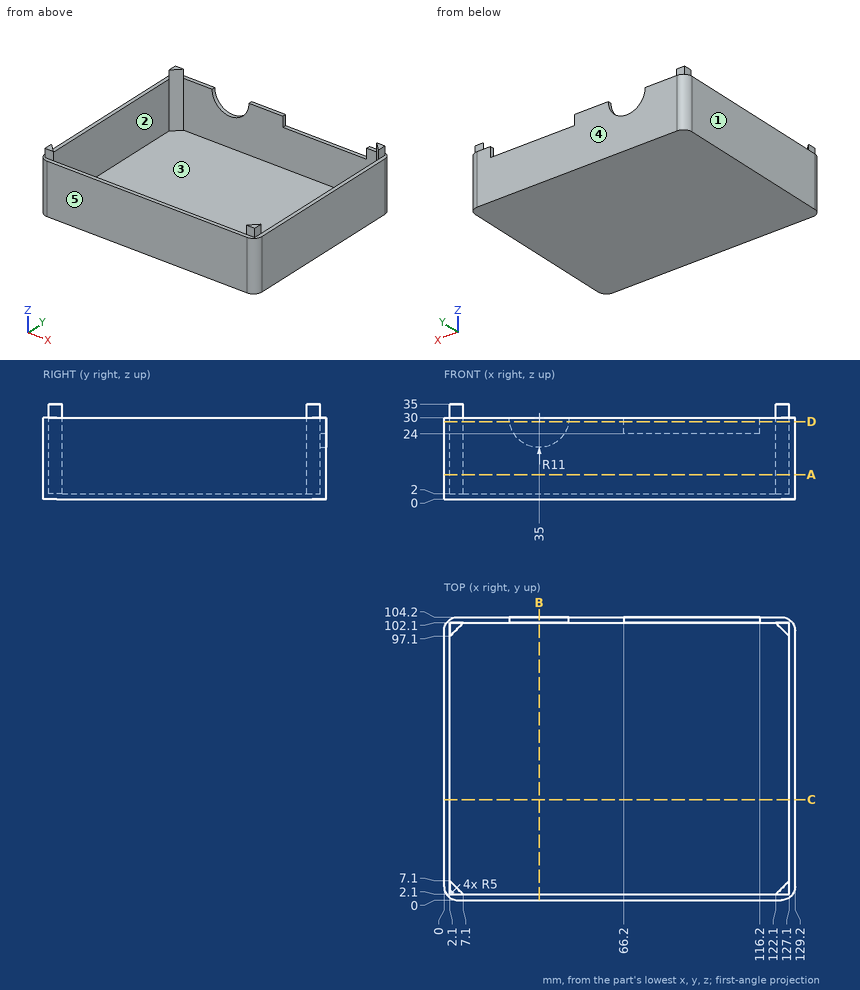
Study the drawing (mm; zero at the part's minimum x, y, z) and answer. A direction names the side the tool comes from. Give positions to 0.01 mm unless a question says otherwise; leave off trailing zeros. Write each loop counter-clockwise with the first axis right and the second up, starting at its lowest first coordinate (ties: lowest second). Pieces come first, ordered by that corner, then holes. Notation, with made-up numbers: (-26, 0) -> (-10, 0) arc R25 cw to (-10, 21) -> close; hole circle Ø3 at (-30.5, 35.25). An arc over 180 degrees is marked (long way). Answer as a JSON object with one key per item and string values. Group by question number.
1) Consider L1, parallel to X at y = 55.5, z = 11; L2, parallel to Y at x = 73, z = 19.5; L3, parallel to Z at x = 58.5, y = 5. Determine where each line is inside the solid, lowest interval first. Write a range as from..to.
2) Each of these flat-tipped pins is pushed along its axis until it touches: P1, Ø1.7, axis at x = 51.5, y = 103, coming from the +Z side; P2, Ø1.5, axis at x = 5, z = 32.5, coming from the +Y side; P3, Ø2.5, axis at y = 100.5, z = 33.5, coming from the +X side. Where does it stop, or does it pass through?
3) Find section B-B (x = 35). Write down the section's boundary in (y, z), and give its area (3 significant figures).
4) The mould has two halves that part along Y. Classify the marked faces 3, 4 and 5: +Y half, -Y half, draft (parallel to the pull), parting line (faces both ways), or undercut.
5) Find section A-A (z = 9). Write down the section's boundary in (x, y), and give its area (3 significant figures).
6) A tool of negligible diameter and unlimited length cuts with its end or side. For the marked faces 1 and 2, from which of +Z, -Z, +X, -X, +Y, -Y can it reach the whole face along a straight path? Write none if from no direction.
7) Find section D-D (z = 28.5). Write down the section's boundary in (x, y), and give its area (3 significant figures).
8) Find section C-C (y = 37). Write down the section's boundary in (x, z), and give its area (3 significant figures).
Values follow:
{
 "1": {"L1": "x = 0..2.1, 127.1..129.2", "L2": "y = 0..2.1, 102.1..104.2", "L3": "z = 0..2"},
 "2": {"P1": "stops at z = 30", "P2": "stops at y = 102.1", "P3": "stops at x = 127.1"},
 "3": {"outline": "(0, 0) -> (104.2, 0) -> (104.2, 19) -> (102.1, 19) -> (102.1, 2) -> (2.1, 2) -> (2.1, 30) -> (0, 30) -> close", "area": "303 mm2"},
 "4": {"face 3": "undercut", "face 4": "+Y half", "face 5": "-Y half"},
 "5": {"outline": "(0, 5) arc R5 ccw to (5, 0) -> (124.2, 0) arc R5 ccw to (129.2, 5) -> (129.2, 99.2) arc R5 ccw to (124.2, 104.2) -> (5, 104.2) arc R5 ccw to (0, 99.2) -> close; hole (2.1, 7.1) -> (7.1, 2.1) -> (122.1, 2.1) -> (127.1, 7.1) -> (127.1, 97.1) -> (122.1, 102.1) -> (7.1, 102.1) -> (2.1, 97.1) -> close", "area": "991 mm2"},
 "6": {"face 1": "+Z, -Z, -X, +Y, -Y", "face 2": "+Z"},
 "7": {"outline": "(0, 5) arc R5 ccw to (5, 0) -> (124.2, 0) arc R5 ccw to (129.2, 5) -> (129.2, 99.2) arc R5 ccw to (124.2, 104.2) -> (116.2, 104.2) -> (116.2, 102.1) -> (122.1, 102.1) -> (127.1, 97.1) -> (127.1, 7.1) -> (122.1, 2.1) -> (7.1, 2.1) -> (2.1, 7.1) -> (2.1, 97.1) -> (7.1, 102.1) -> (24.1, 102.1) -> (24.1, 104.2) -> (5, 104.2) arc R5 ccw to (0, 99.2) -> close; (45.9, 102.1) -> (66.2, 102.1) -> (66.2, 104.2) -> (45.9, 104.2) -> close", "area": "840 mm2"},
 "8": {"outline": "(0, 0) -> (129.2, 0) -> (129.2, 30) -> (127.1, 30) -> (127.1, 2) -> (2.1, 2) -> (2.1, 30) -> (0, 30) -> close", "area": "376 mm2"}
}
